Check sheet for the modelled part. Datum: model origin and axes. Units: mm. A direction names the side the tool comes from. Round coordinates to 2 decimals unless told otherwise and drop trailing zeros. Write each loop counter-clockwise with the first axis right and the second up, starting at its lowest first coordinate (ties: lowest second). Pieces come first, ordered by that corner, then holes. Notation, with made-up numbers: (51.5, -21) -> (86.5, -21) arc R14 cw to (86.5, -1) -> close; hole circle Ø2 at (0, 42). An arc over 180 degrees is marked (long way). Use one line per item in the form item = value. Start each with the question number.
```python
from build123d import *

# Parameters (mm, degrees)
SKETCH001_R  = 4
POCKET_DEPTH = 80.001
CHAMFER_SIZE = 10
FILLET_R     = 4
FILLET001_R  = 2


with BuildPart() as part:
    # Sketch → Revolution (revolve)
    with BuildSketch(Plane.XY):
        Polygon((5, 60), (5, 20), (15, 20), (15, 15), (5, 15), (5, 0), (0, 0), (0, 80), (15, 80), align=None)
    revolve(axis=Axis((0, 0, 0), (0, 1, 0)))

    # Sketch001 (on Face7 of Revolution) → Pocket (cut, through all)
    with BuildSketch(Plane(origin=(0, 80, 0), x_dir=(-1, 0, 0), z_dir=(0, 1, 0))):
        Circle(SKETCH001_R)
    extrude(amount=-POCKET_DEPTH, mode=Mode.SUBTRACT)

    # Chamfer
    chamfer_edges = [part.edges().sort_by_distance(p)[0] for p in [
        (4, 80, 0),
    ]]
    chamfer(chamfer_edges, length=CHAMFER_SIZE)

    # Fillet
    fillet_edges = [part.edges().sort_by_distance(p)[0] for p in [
        (-15, 20, 0),
    ]]
    fillet(fillet_edges, radius=FILLET_R)

    # Fillet001
    fillet001_edges = [part.edges().sort_by_distance(p)[0] for p in [
        (14, 80, 0),
    ]]
    fillet(fillet001_edges, radius=FILLET001_R)


solid = part.part
```
1. Sectioned sample at A-A (z = 0). Enter the section's corners in (x, y), and give its area (3 significant figures).
2. Sectioned sample at C-C (y = 49). Enter the section's corners in (x, z).
3. Sectioned sample at B-B (x = 0). Enter the section's corners in (y, z).
4. Depth check by flat-ended pin: pin 1 (1.5 mm diameter, centred on y = 58.5, z = -5, fed in from +X); pin 2 (1 mm diameter, centred on x = 10, z = 9, fed in from -Y); pin 3 (11 mm diameter, centred on x = 2, z = -1, fed in from +Y). Enter the tip coordinate at first touch or a pass-through.
5. Tool access check on faces 1 (the face through (-14.985, 15.493, -0.66)), 2 (the face through (-1.08, 39.72, 4.88)), 3 (the face through (-4, 15, -4)). Record the directions out of +Z, -Z, +X, -X, +Y, -Y that give a thin tool (end or side, any length) a straight path to the whole face; none if there is none.
6. Mould release check, pull along X, two halves, no side actions. Record for faces 4 (the face through (-2.057, 70.457, -3.954)), 5 (the face through (-2, 20, 5)), 6 (the face through (-1.003, 65.416, -7.642)): +X half, -X half, draft (parallel to the pull), parting line (faces both ways), or undercut.
7. Scan lines: probe 1 along Z at (x, y) = (0, 56.5); probe 2 along Y at (x, z) = (3.5, 6.5); probe 3 along Y at (x, z) = (8, 9). Record each from-to range of solid material in increasing order.
Returned:
q1.outline = (-15, 15) -> (-5, 15) -> (-5, 0) -> (-4, 0) -> (-4, 70) -> (-13.41, 79.41) arc R2 ccw to (-14.83, 80) -> (-15, 80) -> (-5, 60) -> (-5, 20) -> (-11, 20) arc R4 ccw to (-15, 16) -> close; (4, 0) -> (5, 0) -> (5, 15) -> (15, 15) -> (15, 16) arc R4 ccw to (11, 20) -> (5, 20) -> (5, 60) -> (15, 80) -> (14.83, 80) arc R2 ccw to (13.41, 79.41) -> (4, 70) -> close
q1.area = 353 mm^2
q2.outline = circle Ø10 at (0, 0); hole circle Ø8 at (0, 0)
q3.outline = (0, -5) -> (15, -5) -> (15, -15) -> (16, -15) arc R4 ccw to (20, -11) -> (20, -5) -> (60, -5) -> (80, -15) -> (80, -14.83) arc R2 ccw to (79.41, -13.41) -> (70, -4) -> (0, -4) -> close; (0, 4) -> (70, 4) -> (79.41, 13.41) arc R2 ccw to (80, 14.83) -> (80, 15) -> (60, 5) -> (20, 5) -> (20, 11) arc R4 ccw to (16, 15) -> (15, 15) -> (15, 5) -> (0, 5) -> close
q4.pin_1 = 2.63
q4.pin_2 = 15
q4.pin_3 = 73.74
q5.face_1 = +Y, -Y
q5.face_2 = none
q5.face_3 = -Y
q6.face_4 = undercut
q6.face_5 = draft
q6.face_6 = parting line
q7.probe_1 = -5 to -4, 4 to 5
q7.probe_2 = 15 to 20, 64.76 to 73.38
q7.probe_3 = 15 to 19.86, 74.08 to 78.04
